from build123d import *

# Parameters (mm, degrees)
F0_W     = 50
F0_H     = 50
F1_DEPTH = 50
F3_DEPTH = 50.001
F5_DEPTH = 50.001
F7_DEPTH = 50.001
F8_R     = 4.99999


# Not quite as in the source:
# - a fillet or chamfer is up to 0.001 mm smaller than in the source, because OpenCascade refuses the exact size


with BuildPart() as f1:
    # F0 (on Top) → F1 (new body)
    with BuildSketch(Plane.XY):
        Rectangle(F0_W, F0_H)
    extrude(amount=F1_DEPTH)

    # F2 (on face) → F3 (cut, through all)
    with BuildSketch(Plane.XY.offset(50)):
        with BuildLine():
            ThreePointArc((20, 10), (17.0710678119, 17.0710678119), (10, 20))
            Line((10, 20), (-10, 20))
            ThreePointArc((-10, 20), (-17.0710678119, 17.0710678119), (-20, 10))
            Line((-20, 10), (-20, -10))
            ThreePointArc((-20, -10), (-17.0710678119, -17.0710678119), (-10, -20))
            Line((-10, -20), (10, -20))
            ThreePointArc((10, -20), (17.0710678119, -17.0710678119), (20, -10))
            Line((20, -10), (20, 10))
        make_face()
    extrude(amount=-F3_DEPTH, mode=Mode.SUBTRACT)

    # F4 (on face) → F5 (cut, through all)
    with BuildSketch(Plane(origin=(-25, 0, 0), x_dir=(0, -1, 0), z_dir=(-1, 0, 0))):
        with BuildLine():
            Line((10, 45), (-10, 45))
            ThreePointArc((-10, 45), (-17.0710678119, 42.0710678119), (-20, 35))
            Line((-20, 35), (-20, 15))
            ThreePointArc((-20, 15), (-17.0710678119, 7.9289321881), (-10, 5))
            Line((-10, 5), (10, 5))
            ThreePointArc((10, 5), (17.0710678119, 7.9289321881), (20, 15))
            Line((20, 15), (20, 35))
            ThreePointArc((20, 35), (17.0710678119, 42.0710678119), (10, 45))
        make_face()
    extrude(amount=-F5_DEPTH, mode=Mode.SUBTRACT)

    # F6 (on face) → F7 (cut, through all)
    with BuildSketch(Plane.XZ.offset(25)):
        with BuildLine():
            Line((10, 45), (-10, 45))
            ThreePointArc((-10, 45), (-17.0710678119, 42.0710678119), (-20, 35))
            Line((-20, 35), (-20, 15))
            ThreePointArc((-20, 15), (-17.0710678119, 7.9289321881), (-10, 5))
            Line((-10, 5), (10, 5))
            ThreePointArc((10, 5), (17.0710678119, 7.9289321881), (20, 15))
            Line((20, 15), (20, 35))
            ThreePointArc((20, 35), (17.0710678119, 42.0710678119), (10, 45))
        make_face()
    extrude(amount=-F7_DEPTH, mode=Mode.SUBTRACT)

    # F8 (radius 5 in the source; OpenCascade refuses exactly that, so slightly less here)
    f8_edges = [f1.edges().sort_by_distance(p)[0] for p in [
        (0, 25, 0),
        (-25, 0, 0),
        (0, -25, 0),
        (25, 0, 0),
        (25, 25, 25),
        (-25, 25, 25),
        (-25, -25, 25),
        (0, 25, 50),
        (-25, 0, 50),
        (0, -25, 50),
        (25, 0, 50),
        (25, -25, 25),
    ]]
    fillet(f8_edges, radius=F8_R)


solid = f1.part
Verification items for the finished model (mm, model axes). A direction names the side the tool comes from. Coordinates: 2 decimals unless noted, no trailing zeros. Write each loop counter-clockwise with the first axis right and the second up, starting at its lowest first coordinate (ties: lowest second). Pieces come first, ordered by that corner, then holes. Notation, with made-up numbers: (-29, -3.75) - (26, -3.75) arc R20 ccw to (26, 23.25) - close; hole circle Ø5 at (34.5, -35). An arc over 180 degrees is marked (long way). Answer as a JSON object with one key per item and string values.
(1) Cross-section at A-A on x = 1. Give the number of separate pieces and of enclosed holes in the cut face, plus the area to 3 significant figures.
Report:
{"separate pieces": "4", "enclosed holes": "0", "area": "78.5 mm^2"}
(2) Thickness scan on line 1 along X through (y, z) = (-3.5, 46.5); line 2 along Y through (x, z) = (22, 31.5); line 3 along Y through (x, z) = (-22, 37.5). Record the ranges inside material, lowest first.
Report:
{"line 1": "-24.77 to -20, 20 to 24.77", "line 2": "-24.58 to -20, 20 to 24.58", "line 3": "-24.58 to -19.68, 19.68 to 24.58"}
(3) Cross-section at D-D on y = -22. Record the cut outline in (x, z).
Report:
{"outline": "(-24.58, 5) arc R4.58 ccw to (-20, 0.42) - (20, 0.42) arc R4.58 ccw to (24.58, 5) - (24.58, 45) arc R4.58 ccw to (20, 49.58) - (-20, 49.58) arc R4.58 ccw to (-24.58, 45) - close; hole (-20, 15) arc R10 ccw to (-10, 5) - (10, 5) arc R10 ccw to (20, 15) - (20, 35) arc R10 ccw to (10, 45) - (-10, 45) arc R10 ccw to (-20, 35) - close"}
(4) Mould release check, pull along Y, two halves, no side actions. Record for faces 5 (the flat face through (0, 22, 5)), 6 (the cylindrical face through (21.86, 17.15, 8.01)), 7 (the cylindrical face through (-24, 23, 25)), 8 (the flat face through (-20, 0, 48)): pulls with the +Y half, pulls with the -Y half, needs draft (parallel to the pull), parting line crosses it, or undercut.
Report:
{"face 5": "needs draft", "face 6": "undercut", "face 7": "pulls with the +Y half", "face 8": "undercut"}
(5) Gauge pin test, flat ends, axial feed: pin 1 Ø1.5 at (x, z) = (-2, 3.5) entering from +Y; pin 2 Ø5.5 at (y, z) = (1.5, 2) entering from +X; pin 3 Ø1.5 at (x, y) = (-22.5, 2) entering from -Z; pin 4 Ø6 at (x, z) = (4.5, 43.5) entering from -Y. Record the tip position at first contact, or that the pin passes through.
Report:
{"pin 1": "y = 24.94", "pin 2": "x = 24.99", "pin 3": "z = 0.32", "pin 4": "y = -25"}
(6) Cross-section at C-C on y = 18. Record the cut outline in (x, z), plus the area to 3 significant figures.
Report:
{"outline": "(-25, 5) arc R5 ccw to (-20, 0) - (-16, 0) - (-16, 7) arc R10 cw to (-18, 9) - (-25, 9) - close; (-25, 41) - (-18, 41) arc R10 cw to (-16, 43) - (-16, 50) - (-20, 50) arc R5 ccw to (-25, 45) - close; (16, 0) - (20, 0) arc R5 ccw to (25, 5) - (25, 9) - (18, 9) arc R10 cw to (16, 7) - close; (16, 43) arc R10 cw to (18, 41) - (25, 41) - (25, 45) arc R5 ccw to (20, 50) - (16, 50) - close", "area": "294 mm^2"}
(7) Tool access check on faces 1 (the flat face through (-25, -16.4, 7.1)), 2 (the cylindrical face through (16.99, -17.15, 46.97)), 3 (the flat face through (0, -23, 5)), 4 (the flat face through (22, 0, 45)). Record the directions out of +Z, -Z, +X, -X, +Y, -Y that give a thin tool (end or side, any length) a straight path to the whole face; none if there is none.
Report:
{"face 1": "+Z, -Z, -X, +Y, -Y", "face 2": "+Z, -Z", "face 3": "+Y, -Y", "face 4": "+X, -X"}
